from build123d import *

# Parameters (mm, degrees)
SKETCH_1_W          = 32
SKETCH_1_H          = 46
EXTRUDE_1_DEPTH     = 3
SKETCH_2_R          = 4.1
SKETCH_2_R_2        = 1.4
CUT_EXTRUDE_1_DEPTH = 4
SKETCH_3_R          = 1.7
CUT_EXTRUDE_2_DEPTH = 4


with BuildPart() as part:
    # 草图1 → 凸台-拉伸1 (new body)
    with BuildSketch(Plane.XY):
        Rectangle(SKETCH_1_W, SKETCH_1_H)
    extrude(amount=-EXTRUDE_1_DEPTH)

    # 草图2 → 切除-拉伸1 (cut)
    with BuildSketch(Plane.XY):
        Circle(SKETCH_2_R)
        with Locations((9.6, 0)):
            Circle(SKETCH_2_R_2)
    extrude(amount=-CUT_EXTRUDE_1_DEPTH, mode=Mode.SUBTRACT)

    # 草图3 → 切除-拉伸2 (cut)
    with BuildSketch(Plane.XY):
        with Locations((-11, 15)):
            Circle(SKETCH_3_R)
        with Locations((11, 15)):
            Circle(SKETCH_3_R)
    extrude(amount=-CUT_EXTRUDE_2_DEPTH, mode=Mode.SUBTRACT)


solid = part.part
Could you check a few things on this model? Use its own coordinates, in mm. Give positions to 0.01 mm unless a question says otherwise; leave off trailing zeros. Write each loop counter-clockwise with the first axis right and the second up, starting at its lowest first coordinate (ties: lowest second). Pieces come first, ordered by that corner, then holes. Notation, with made-up numbers: (1.5, 79) -> (18.5, 79) arc R17 cw to (18.5, 93) -> close; hole circle Ø1 at (53.5, -24). An arc over 180 degrees is marked (long way). Answer as CSV lines item,"result". Start each with the question number.
(1) If we section it at D-D, the plane y = 0: Write out the boundary of the cut face in (x, z).
(2) If we section it at C-C, the plane z = -0.6: Write out the boundary of the cut face in (x, y), and give its area (3 significant figures).
(3) Please list where these lines run through material, in increasing order: line 1 (X direction, y = 14, z = -1.95); line 2 (X direction, y = -1, z = -2); line 3 (Y direction, x = 0, z = -0.55).
(4) If we section it at A-A, the plane y = 15: Write out the boundary of the cut face in (x, z).
(5) If we mould it in two halves opening along Y, with no side actions, what happens to faces 1 (the face through (0, 23, -1)), 2 (the face through (-0.534, 4.065, -1.479)), 3 (the face through (11, 0, -1)), 4 (the face through (-16, 0, -1))? For each: +Y half, -Y half, draft (parallel to the pull), parting line (faces both ways), or undercut.
(6) I'm going to push a flat-ended pin straight in: pin 1 Ø2 at (x, y) = (-11, 15) entering from +Z. Where does the tip first touch, or does it pass through?
(7) If we section it at B-B, the plane x = -11: Write out the boundary of the cut face in (y, z).
Answer list:
1,outline,"(-16, -3) -> (-4.1, -3) -> (-4.1, 0) -> (-16, 0) -> close; (4.1, -3) -> (8.2, -3) -> (8.2, 0) -> (4.1, 0) -> close; (11, -3) -> (16, -3) -> (16, 0) -> (11, 0) -> close"
2,outline,"(-16, -23) -> (16, -23) -> (16, 23) -> (-16, 23) -> close; hole circle Ø3.4 at (-11, 15); hole circle Ø8.2 at (0, 0); hole circle Ø2.8 at (9.6, 0); hole circle Ø3.4 at (11, 15)"
2,area,"1,390 mm^2"
3,line 1,"-16 to -12.37, -9.63 to 9.63, 12.37 to 16"
3,line 2,"-16 to -3.98, 3.98 to 8.62, 10.58 to 16"
3,line 3,"-23 to -4.1, 4.1 to 23"
4,outline,"(-16, -3) -> (-12.7, -3) -> (-12.7, 0) -> (-16, 0) -> close; (-9.3, -3) -> (9.3, -3) -> (9.3, 0) -> (-9.3, 0) -> close; (12.7, -3) -> (16, -3) -> (16, 0) -> (12.7, 0) -> close"
5,face 1,"+Y half"
5,face 2,"undercut"
5,face 3,"undercut"
5,face 4,"draft"
6,pin 1,"through"
7,outline,"(-23, -3) -> (13.3, -3) -> (13.3, 0) -> (-23, 0) -> close; (16.7, -3) -> (23, -3) -> (23, 0) -> (16.7, 0) -> close"
